from build123d import *

# Parameters (mm, degrees)
SKETCH1_R           = 7.15
BOSS_EXTRUDE1_DEPTH = 43
SKETCH2_R           = 5
CUT_EXTRUDE1_DEPTH  = 0.1
SKETCH3_R           = 0.75
BOSS_EXTRUDE2_DEPTH = 5
FILLET1_R           = 0.25


with BuildPart() as part:
    # Sketch1 → Boss-Extrude1 (new body)
    with BuildSketch(Plane.XY):
        Circle(SKETCH1_R)
    extrude(amount=BOSS_EXTRUDE1_DEPTH)

    # Sketch2 → Cut-Extrude1 (cut)
    with BuildSketch(Plane(origin=(0, 0, 0), x_dir=(-1, 0, 0), z_dir=(0, 0, -1))):
        Circle(SKETCH2_R)
    extrude(amount=-CUT_EXTRUDE1_DEPTH, mode=Mode.SUBTRACT)

    # Sketch3 → Boss-Extrude2 (add)
    with BuildSketch(Plane.XY.offset(43)):
        with Locations((0, 4)):
            Circle(SKETCH3_R)
        with Locations((1.735534956, 3.603875472)):
            Circle(SKETCH3_R)
        with Locations((3.12732593, 2.493959207)):
            Circle(SKETCH3_R)
        with Locations((3.899711649, 0.890083736)):
            Circle(SKETCH3_R)
        with Locations((3.899711649, -0.890083736)):
            Circle(SKETCH3_R)
        with Locations((3.12732593, -2.493959207)):
            Circle(SKETCH3_R)
        with Locations((1.735534956, -3.603875472)):
            Circle(SKETCH3_R)
        with Locations((0, -4)):
            Circle(SKETCH3_R)
        with Locations((-1.735534956, -3.603875472)):
            Circle(SKETCH3_R)
        with Locations((-3.12732593, -2.493959207)):
            Circle(SKETCH3_R)
        with Locations((-3.899711649, -0.890083736)):
            Circle(SKETCH3_R)
        with Locations((-3.899711649, 0.890083736)):
            Circle(SKETCH3_R)
        with Locations((-3.12732593, 2.493959207)):
            Circle(SKETCH3_R)
    extrude(amount=BOSS_EXTRUDE2_DEPTH)

    # Fillet1
    fillet1_edges = [part.edges().sort_by_distance(p)[0] for p in [
        (-7.15, 0, 0),
        (-7.15, 0, 43),
    ]]
    fillet(fillet1_edges, radius=FILLET1_R)


solid = part.part
The model under review builds one solid part; all positions refer to its coordinate system, in mm. A direction names the side the tool comes from. Round coordinates to 2 decimals unless told otherwise and drop trailing zeros. Order: outer loops, then holes, each group sorted by start corner. A loop starts at its lowest first (then second) coordinate and runs counter-clockwise, first axis right, second up. Notation, with made-up numbers: (41, -5) -> (62, -5) arc R35 ccw to (62, 27) -> close; hole circle Ø8 at (52, 16.5). An arc over 180 degrees is marked (long way). Return JSON: item names as keys, results as strings.
1. For faces 1 (the face through (0, 0, 0.1)), 2 (the face through (5, 2, 0)), 3 (the face through (0, 0, 43)), list the 3-axis set-ups (+Z, -Z, +X, -X, +Y, -Y) from which the entire face can be reached by the end or side of a thin tool; tool diameter is ignored.
Answer block:
{"face 1": "-Z", "face 2": "-Z, +X, -X, +Y, -Y", "face 3": "+Z"}
2. The part is to be moulded in two halves that separate along X. For faces 4 (the face through (3.82, -2.78, 45.46)), 5 (the face through (-2.435, -2.781, 45.465)), 6 (the face through (2, 4, 48)), say which applies: +X half, -X half, draft (parallel to the pull), parting line (faces both ways), or undercut.
Answer block:
{"face 4": "undercut", "face 5": "undercut", "face 6": "draft"}
3. Insertion check: P1, Ø5, axis at x = 1.5, y = 0, coming from the -Z side; P2, Ø2, axis at x = -2, z = 35, coming from the -Y side; P3, Ø8, axis at y = -5.5, z = 9.5, coming from the -X side. Each pin has a flat end and moves straight along its axis. Give the tip position at first contact, or say it passes through.
Answer block:
{"P1": "stops at z = 0.1", "P2": "stops at y = -7.08", "P3": "stops at x = -6.99"}
4. Take a section at A-A (x = 0). Write out the cut boundary in (y, z), then the cut area to 3 significant figures.
Answer block:
{"outline": "(-7.15, 0.25) arc R0.25 ccw to (-6.9, 0) -> (-5, 0) -> (-5, 0.1) -> (5, 0.1) -> (5, 0) -> (6.9, 0) arc R0.25 ccw to (7.15, 0.25) -> (7.15, 42.75) arc R0.25 ccw to (6.9, 43) -> (4.75, 43) -> (4.75, 48) -> (3.25, 48) -> (3.25, 43) -> (-3.25, 43) -> (-3.25, 48) -> (-4.75, 48) -> (-4.75, 43) -> (-6.9, 43) arc R0.25 ccw to (-7.15, 42.75) -> close", "area": "629 mm²"}
5. Take a section at B-B (z = 18). Write out the cut boundary in (x, y), then the cut area to 3 significant figures.
Answer block:
{"outline": "circle Ø14.3 at (0, 0)", "area": "161 mm²"}
6. For L1, parallel to Z at x = 5.5, y = -2; L2, parallel to Z at x = 1.5, y = -1.25; L3, parallel to Y at x = 0.25, z = 33.5, list the stretches that pass through material, from the lowest coordinate up. Write a range as [from, to].
Answer block:
{"L1": "z = [0, 43]", "L2": "z = [0.1, 43]", "L3": "y = [-7.15, 7.15]"}
